Can you work these out from the model? Positions are in its coordinate system, mm. Round coordinates to 2 decimals unless told otherwise and drop trailing zeros. Loops run counter-clockwise (first coordinate to the right, second up) from the corner with the lowest first, then second, coordinate; pieces in that order, holes last. Notation, with made-up numbers: (63.5, 23.25) -> (84.5, 23.25) arc R15 cw to (84.5, 34.25) -> close; hole circle Ø11 at (-39, 30). An arc over 180 degrees is marked (long way). Use a Markdown table: item, result.
from build123d import *

# Parameters (mm, degrees)
F1_DEPTH = 0.5
F2_R     = 6.35
F3_DEPTH = 12.7
F4_W     = 10.370853
F4_H     = 5.103117
F5_DEPTH = 12.7


with BuildPart() as f1:
    # F0 (on Front) → F1 (new body, symmetric)
    with BuildSketch(Plane.XZ):
        Polygon((-43.18, 43.18), (0, 0), (33.02, 0), (33.02, 43.18), align=None)
    extrude(amount=F1_DEPTH, both=True)

    # F2 (on Front) → F3 (cut, symmetric)
    with BuildSketch(Plane.XZ):
        with Locations((22.86, 30.48)):
            Circle(F2_R)
    extrude(amount=F3_DEPTH, both=True, mode=Mode.SUBTRACT)

    # F4 (on Front) → F5 (cut, symmetric)
    with BuildSketch(Plane.XZ):
        with Locations((-13.880418, 33.682564)):
            Rectangle(F4_W, F4_H)
    extrude(amount=F5_DEPTH, both=True, mode=Mode.SUBTRACT)


solid = f1.part
1. Will these pins go through, and if not, where does the flat tip stop? pin 1 Ø0.5 at (y, z) = (0, 34.5) entering from -X; pin 2 Ø7.5 at (x, z) = (22.86, 30.48) entering from +Y.
Answer sheet:
| item | result |
|---|---|
| pin 1 | stops at x = -34.75 |
| pin 2 | passes through |
2. I want a section at D-D (x = -7). Please give me the cut outline in (y, z), plus the area to 3 significant figures.
Answer sheet:
| item | result |
|---|---|
| outline | (-0.5, 7) -> (0.5, 7) -> (0.5, 43.18) -> (-0.5, 43.18) -> close |
| area | 36.2 mm² |
3. If we mould it in two halves opening along Z, with no side actions, what happens to faces 1 (the flat face through (3, 0.5, 27)), 2 (the flat face through (-22, 0, 22)), 3 (the cylindrical face through (21.48, -0.01, 24.28))? For each: +Z half, -Z half, draft (parallel to the pull), parting line (faces both ways), or undercut.
Answer sheet:
| item | result |
|---|---|
| face 1 | draft |
| face 2 | -Z half |
| face 3 | undercut |
4. I want a section at B-B (y = 0.15). Please give me the cut outline in (x, z) (3 decimals).
Answer sheet:
| item | result |
|---|---|
| outline | (-43.18, 43.18) -> (0, 0) -> (33.02, 0) -> (33.02, 43.18) -> close; hole (-19.066, 31.131) -> (-8.695, 31.131) -> (-8.695, 36.234) -> (-19.066, 36.234) -> close; hole circle Ø12.7 at (22.86, 30.48) |
5. I need wall thicknesses on line 1 (Z direction, x = 22.86, y = 0); line 2 (X direction, y = 0.4, z = 34.5) (1 decimal); line 3 (X direction, y = 0.2, z = 31.5) (3 decimals). Which ranges of each line are inside material? Lowest first, please.
Answer sheet:
| item | result |
|---|---|
| line 1 | z = 0 to 24.13, 36.83 to 43.18 |
| line 2 | x = -34.5 to -19.1, -8.7 to 17.9, 27.8 to 33 |
| line 3 | x = -31.5 to -19.066, -8.695 to 16.592, 29.128 to 33.02 |
6. I want a section at A-A (x = 22.86). Please give me the cut outline in (y, z).
Answer sheet:
| item | result |
|---|---|
| outline | (-0.5, 0) -> (0.5, 0) -> (0.5, 24.13) -> (-0.5, 24.13) -> close; (-0.5, 36.83) -> (0.5, 36.83) -> (0.5, 43.18) -> (-0.5, 43.18) -> close |
7. I want a section at C-C (z = 35). Please give me the cut outline in (x, y) (3 decimals).
Answer sheet:
| item | result |
|---|---|
| outline | (-35, -0.5) -> (-19.066, -0.5) -> (-19.066, 0.5) -> (-35, 0.5) -> close; (-8.695, -0.5) -> (18.4, -0.5) -> (18.4, 0.5) -> (-8.695, 0.5) -> close; (27.32, -0.5) -> (33.02, -0.5) -> (33.02, 0.5) -> (27.32, 0.5) -> close |
